For this review, take the finished solid that the model builds, in its own axes (mm). Give positions to 0.01 mm unless a question says otherwise; leave off trailing zeros.
1) We need section A-A on y = 0.7. Give the number of separate pieces and of enclosed holes in the cut face, and give its area (3 significant figures).
2) For P1, Ø9, axis at x = 55.5, z = 62.5, coming from the +Y side, flat-tipped, find the tip position at first contact; note if it passes through.
3) Wall thickness on line 1 along Z through (x, y) = (351.5, 0.5); line 2 along Z through (x, y) = (-428, 0.95): over which ranges is each line inside the solid? List them lowest first.
Autodesk Inventor part; units mm, degrees
ref_plane "YZ Plane" through (0, 0, 0) normal (1, 0, 0) x (0, 1, 0)
ref_plane "XZ Plane" through (0, 0, 0) normal (0, 1, 0) x (-1, 0, 0)
ref_plane "XY Plane" through (0, 0, 0) normal (0, 0, 1) x (1, 0, 0)
sketch "Skin Scheme" plane through (0, 0, 0) normal (0, 1, 0) x (-1, 0, 0)
  line L0 (547.5, -84.5) -> (-547.5, -84.5)
  line L1 (-547.5, -84.5) -> (-547.5, 84.5)
  line L2 (-547.5, 84.5) -> (547.5, 84.5)
  line L3 (547.5, 84.5) -> (547.5, -84.5)
  circle A0 centre (425.5, -62.5) radius 5
  circle A1 centre (388.5, -62.5) radius 5
  circle A2 centre (351.5, -62.5) radius 5
  circle A3 centre (314.5, -62.5) radius 5
  circle A4 centre (277.5, -62.5) radius 5
  circle A5 centre (240.5, -62.5) radius 5
  circle A6 centre (203.5, -62.5) radius 5
  circle A7 centre (166.5, -62.5) radius 5
  circle A8 centre (129.5, -62.5) radius 5
  circle A9 centre (92.5, -62.5) radius 5
  circle A10 centre (55.5, -62.5) radius 5
  circle A11 centre (18.5, -62.5) radius 5
  circle A12 centre (-18.5, -62.5) radius 5
  circle A13 centre (-55.5, -62.5) radius 5
  circle A14 centre (-92.5, -62.5) radius 5
  circle A15 centre (-129.5, -62.5) radius 5
  circle A16 centre (-166.5, -62.5) radius 5
  circle A17 centre (-203.5, -62.5) radius 5
  circle A18 centre (425.5, 62.5) radius 5
  circle A19 centre (388.5, 62.5) radius 5
  circle A20 centre (351.5, 62.5) radius 5
  circle A21 centre (314.5, 62.5) radius 5
  circle A22 centre (277.5, 62.5) radius 5
  circle A23 centre (240.5, 62.5) radius 5
  circle A24 centre (203.5, 62.5) radius 5
  circle A25 centre (166.5, 62.5) radius 5
  circle A26 centre (129.5, 62.5) radius 5
  circle A27 centre (92.5, 62.5) radius 5
  circle A28 centre (55.5, 62.5) radius 5
  circle A29 centre (18.5, 62.5) radius 5
  circle A30 centre (-18.5, 62.5) radius 5
  circle A31 centre (-55.5, 62.5) radius 5
  circle A32 centre (-92.5, 62.5) radius 5
  circle A33 centre (-129.5, 62.5) radius 5
  circle A34 centre (-166.5, 62.5) radius 5
  circle A35 centre (-203.5, 62.5) radius 5
  circle A36 centre (-240.5, -62.5) radius 5
  circle A37 centre (-240.5, 62.5) radius 5
  circle A38 centre (-277.5, -62.5) radius 5
  circle A39 centre (-277.5, 62.5) radius 5
  circle A40 centre (-314.5, -62.5) radius 5
  circle A41 centre (-314.5, 62.5) radius 5
  circle A42 centre (-351.5, -62.5) radius 5
  circle A43 centre (-351.5, 62.5) radius 5
  circle A44 centre (-388.5, -62.5) radius 5
  circle A45 centre (-388.5, 62.5) radius 5
  circle A46 centre (-425.5, -62.5) radius 5
  circle A47 centre (-425.5, 62.5) radius 5
  point P0 (0, 0)
  dimension "d0" = 1095
  dimension "d1" = 547.5
  dimension "d2" = 169
  dimension "d3" = 84.5
  dimension "d4" = 10
  dimension "d5" = 122
  dimension "d6" = 22
  dimension "d9" = 37
  dimension "d12" = 125
extrude "Skin Body" add sketch "Skin Scheme" along normal blind 1
sketch "End Cut Outline" plane through (0, 1, 0) normal (0, 1, 0) x (1, 0, 0)
  line L0 (-497.5, 94.5) -> (-557.5, 94.5)
  line L1 (-557.5, 94.5) -> (-557.5, -94.5)
  line L2 (-557.5, -94.5) -> (-497.5, -94.5)
  line L3 (-497.5, -94.5) -> (-497.5, 94.5)
  line L4 (547.5, 84.5) -> (-547.5, 84.5)
  line L5 (-547.5, -84.5) -> (547.5, -84.5)
  line L6 (-547.5, 84.5) -> (-547.5, -84.5)
  point P0 (0, 0)
  dimension "d19" = 10
  dimension "d20" = 10
  dimension "d21" = 10
  dimension "d22" = 50
extrude "End Cut" cut sketch "End Cut Outline" along normal through all both and the other way through all
mirror "End Cut Mirror" about plane through (0, 0, 0) normal (1, 0, 0) of "End Cut"
properties part number "Skin NPS 8 Internal" material "Rubber, Silicone"
Results list:
1. separate pieces: 1
1. enclosed holes: 48
1. area: 164,000 mm2
2. P1: passes through
3. line 1: z = -84.5 to -67.5, -57.5 to 57.5, 67.5 to 84.5
3. line 2: z = -84.5 to -66.83, -58.17 to 58.17, 66.83 to 84.5
